Geometry check sheet. Reference: the model listing, model coordinates, mm. Give positions to 0.01 mm unless a question says otherwise; leave off trailing zeros. Loops run counter-clockwise (first coordinate to the right, second up) from the corner with the lowest first, then second, coordinate; pieces in that order, holes last. Notation, with made-up numbers: (13, 2) -> (61, 2) arc R34 cw to (61, 38) -> close; hole circle Ø3 at (81.5, 0). An arc over 180 degrees is marked (long way). Answer as a JSON object with one key per item and string values.
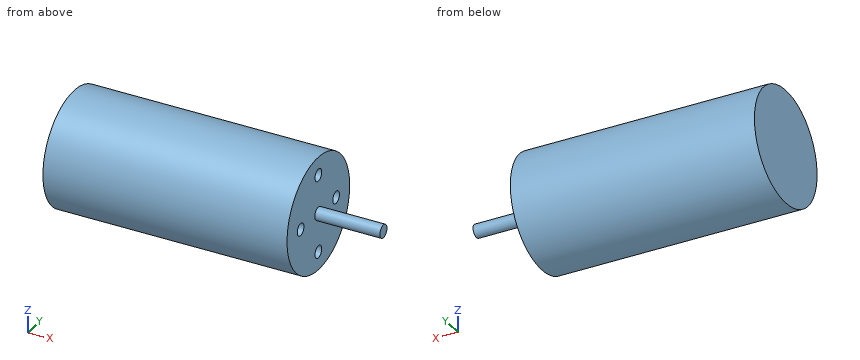
from build123d import *

# Parameters (mm, degrees)
F0_R     = 14
F1_DEPTH = 60
F2_R     = 1.5875
F3_DEPTH = 16
F4_R     = 1.5
F5_DEPTH = 6


with BuildPart() as f1:
    # F0 (on Right) → F1 (new body)
    with BuildSketch(Plane.YZ):
        Circle(F0_R)
    extrude(amount=-F1_DEPTH)

    # F2 (on face) → F3 (join)
    with BuildSketch(Plane.YZ):
        Circle(F2_R)
    extrude(amount=F3_DEPTH)

    # F4 (on face) → F5 (cut)
    with BuildSketch(Plane.YZ):
        with Locations((0, 9.525)):
            Circle(F4_R)
        with Locations((7.9375, 0)):
            Circle(F4_R)
        with Locations((0, -9.525)):
            Circle(F4_R)
        with Locations((-7.9375, 0)):
            Circle(F4_R)
    extrude(amount=-F5_DEPTH, mode=Mode.SUBTRACT)


solid = f1.part
1) Section check D-D on y = -5. Record the cut outline in (x, z).
Geometry check:
{"outline": "(-60, -13.08) -> (0, -13.08) -> (0, 13.08) -> (-60, 13.08) -> close"}
2) Section check B-B on z = 0. Record the cut outline in (x, y), plus the area to 3 significant figures.
Geometry check:
{"outline": "(-60, -14) -> (0, -14) -> (0, -9.44) -> (-6, -9.44) -> (-6, -6.44) -> (0, -6.44) -> (0, -1.59) -> (16, -1.59) -> (16, 1.59) -> (0, 1.59) -> (0, 6.44) -> (-6, 6.44) -> (-6, 9.44) -> (0, 9.44) -> (0, 14) -> (-60, 14) -> close", "area": "1,690 mm2"}
3) Section check A-A on y = 0. Record the cut outline in (x, z) (1 decimal), plus the area to 3 significant figures.
Geometry check:
{"outline": "(-60, -14) -> (0, -14) -> (0, -11) -> (-6, -11) -> (-6, -8) -> (0, -8) -> (0, -1.6) -> (16, -1.6) -> (16, 1.6) -> (0, 1.6) -> (0, 8) -> (-6, 8) -> (-6, 11) -> (0, 11) -> (0, 14) -> (-60, 14) -> close", "area": "1,690 mm2"}
4) Section check C-C on x = -12. Record the cut outline in (y, z).
Geometry check:
{"outline": "circle Ø28 at (0, 0)"}
5) Material ranges on line 1 along Z through (x, y) = (-4.4, 0) (3 decimals); line 2 along X through (y, z) = (-12.5, -2.25); line 3 along Y through (x, z) = (-43.5, 0.25), recorded low to high. Write a range as from..to.
Geometry check:
{"line 1": "z = -14..-11.025, -8.025..8.025, 11.025..14", "line 2": "x = -60..0", "line 3": "y = -14..14"}
6) Depth check by flat-ended pin: P1, Ø3.5, axis at y = 8.5, z = 0.5, coming from the +X side; P2, Ø6, axis at x = -51, z = 8.5, coming from the -Y side; P3, Ø1.5, axis at x = -12, y = -8.5, coming from the -Z side. Enter the tip coordinate at first touch or a pass-through.
Geometry check:
{"P1": "stops at x = 0", "P2": "stops at y = -12.87", "P3": "stops at z = -11.66"}
